Here's how the part is built. I have some questions about the finished solid (model axes, mm). A direction names the side the tool comes from. Coordinates: 2 decimals unless noted, no trailing zeros. Order: outer loops, then holes, each group sorted by start corner. A loop starts at its lowest first (then second) coordinate and runs counter-clockwise, first axis right, second up. Notation, with made-up numbers: M 65,-26 L 78,-26 A17 cw 78,-19 Z; hole C 84,-9.75 d4. An arc over 180 degrees is marked long. One line per question, with ' | ' between items. Start each with the question number.
```python
from build123d import *

# Parameters (mm, degrees)
BOSS_EXTRUDE1_DEPTH     = 36
FILLET1_R               = 12
BOSS_EXTRUDE2_DEPTH     = 8
FILLET2_R               = 15
BOSS_EXTRUDE3_START     = 5
SKETCH3_R               = 15
BOSS_EXTRUDE3_DEPTH     = 5
HOLE1_D                 = 12
M12X1_25_TAPPED_HOLE1_D = 10.8
RIB1_REACH              = 92.255
SKETCH9_WALL_W          = 228.161236354
SKETCH9_WALL_H          = 10


with BuildPart() as part:
    # Sketch1 → Boss-Extrude1 (new, symmetric)
    with BuildSketch(Plane.XY):
        Polygon((0, 0), (0, 6), (5, 6), (5, 10), (35, 10), (35, 0), align=None)
    extrude(amount=BOSS_EXTRUDE1_DEPTH, both=True)

    # Fillet1
    fillet1_edges = [part.edges().sort_by_distance(p)[0] for p in [
        (35, 5, -36),
        (35, 5, 36),
    ]]
    fillet(fillet1_edges, radius=FILLET1_R)

    # Sketch2 → Boss-Extrude2 (add)
    with BuildSketch(Plane.ZY.offset(-5)):
        with BuildLine():
            Line((-15, 60), (-15, 10))
            Line((-15, 10), (15, 10))
            Line((15, 10), (15, 60))
            ThreePointArc((15, 60), (0, 75), (-15, 60))
        make_face()
    extrude(amount=-BOSS_EXTRUDE2_DEPTH)

    # Fillet2
    fillet2_edges = [part.edges().sort_by_distance(p)[0] for p in [
        (9, 10, 15),
        (9, 10, -15),
    ]]
    fillet(fillet2_edges, radius=FILLET2_R)

    # Sketch3 → Boss-Extrude3 (add)
    with BuildSketch(Plane.ZY.offset(-5).offset(BOSS_EXTRUDE3_START)):
        with Locations((0, 60)):
            Circle(SKETCH3_R)
    extrude(amount=-BOSS_EXTRUDE3_DEPTH)

    # Hole1 (through all)
    with Locations(Plane(origin=(13, 0, 0), x_dir=(0, 0, -1), z_dir=(1, 0, 0))):
        with Locations((0, 60)):
            Hole(HOLE1_D / 2)

    # M12x1.25 Tapped Hole1 (through all)
    with Locations(Plane(origin=(0, 10, 0), x_dir=(1, 0, 0), z_dir=(0, 1, 0))):
        with Locations((23, -24), (23, 24)):
            Hole(M12X1_25_TAPPED_HOLE1_D / 2)

    # Sketch9 wall → Rib1 (add, up to next)
    with BuildSketch(Plane(origin=(24, 30, 0), x_dir=(0.481918749772, -0.876215908677, 0), z_dir=(0.876215908677, 0.481918749772, 0)), mode=Mode.PRIVATE) as rib1_sk1:
        Rectangle(SKETCH9_WALL_W, SKETCH9_WALL_H)
    rib1_tool1 = extrude(rib1_sk1.sketch, amount=-RIB1_REACH, mode=Mode.PRIVATE) - part.part
    add(rib1_tool1.solids().sort_by_distance((24, 30, 0))[0])


solid = part.part
```
1. We'd pull the mould along X, two halves only. Please class faces 1 (the face through (35, 5, 0)), 2 (the face through (9.06, 14.28, -19.51)), 3 (the face through (5, 21, 1)), 4 (the face through (17.85, 4.93, 22.38)): released by +X, released by -X, zero draft, split by the parting line, or undercut.
2. I need wall thicknesses on line 1 (Z direction, x = 23, y = 2.5); line 2 (X direction, y = 3, z = -24); line 3 (Y direction, x = 5.75, z = 0). Which ranges of each line are inside material? Lowest first, please.
3. Will these pins go through, and if not, where does the flat tip stop? pin 1 (1.5 mm diameter, centred on x = 5.5, y = 38.5, fed in from +Z); pin 2 (16 mm diameter, centred on y = 46, z = -10, fed in from -X); pin 3 (14 mm diameter, centred on x = 23, z = 24, fed in from +Y); pin 4 (5.5 mm diameter, centred on x = 1.5, z = 12.5, fed in from +Y).
4. Which directions (+Z, -Z, +X, -X, +Y, -Y) give clear straight access to the entire face, cutting with the end or side of a thin tool? Please do faces 5 (the face through (9, 42, 15)), 6 (the face through (13, 43, 6)), 7 (the face through (23, 10, -17)), 8 (the face through (23, 10, 17)), 9 (the face through (2, 6, 1)).
5. Imagine slicing it at A-A (z = 0). List the corners of the cut face in (x, y) for me, then the cut area to 3 significant figures.
6. Imagine slicing it at C-C (z = 9). List the corners of the cut face in (x, y) for me.
7. Imagine slicing it at B-B (x = 24). List the corners of the cut face in (y, z) for me.
8. Imagine slicing it at D-D (y = 20). List the corners of the cut face in (x, z) for me, then the cut area to 3 significant figures.
Entries:
1) face 1: released by +X | face 2: zero draft | face 3: released by -X | face 4: undercut
2) line 1: -36 to -29.4, -18.6 to 18.6, 29.4 to 36 | line 2: 0 to 17.6, 28.4 to 35 | line 3: 0 to 54, 66 to 75
3) pin 1: z = 15 | pin 2: x = 0 | pin 3: y = 10 | pin 4: y = 71.4
4) face 5: +Z, +X, -X, +Y | face 6: +X, +Y | face 7: -Z, +X, +Y | face 8: +Z, +X, +Y | face 9: +Z, -Z, -X
5) outline: M 0,0 L 35,0 L 35,10 L 13,50 L 13,54 L 0,54 L 0,45 L 5,45 L 5,6 L 0,6 Z; M 0,66 L 13,66 L 13,75 L 0,75 Z | area: 1,280 mm²
6) outline: M 0,0 L 35,0 L 35,10 L 13,10 L 13,72 L 0,72 L 0,48 L 5,48 L 5,6 L 0,6 Z
7) outline: M 0,-35.96 L 10,-35.96 L 10,-29.31 L 0,-29.31 Z; M 0,-18.69 L 10,-18.69 L 10,-5 L 30,-5 L 30,5 L 10,5 L 10,18.69 L 0,18.69 Z; M 0,29.31 L 10,29.31 L 10,35.96 L 0,35.96 Z
8) outline: M 5,-15.86 L 13,-15.86 L 13,-5 L 29.5,-5 L 29.5,5 L 13,5 L 13,15.86 L 5,15.86 Z | area: 419 mm²
